Can you work these out from the model? Positions are in its coordinate system, mm. A direction names the side the tool comes from. Coordinates: 2 decimals unless noted, no trailing zeros. Order: outer loops, then holes, each group sorted by start corner. A loop starts at its lowest first (then second) coordinate and runs counter-clockwise, first axis right, second up. Notation, with made-up numbers: (59, -38) -> (109, -38) arc R12 ccw to (109, -21) -> close; hole circle Ø8 at (53, 46.5). An arc over 180 degrees is marked (long way). Answer as CSV lines item,"result".
from build123d import *

# Parameters (mm, degrees)
SKETCH_1_W       = 26.1
SKETCH_1_H       = 45.1
SKETCH_1_R       = 1
EXTRUDE_1_DEPTH  = 1.6
EXTRUDE_2_DEPTH  = 1.8
SKETCH_3_W       = 11
SKETCH_3_H       = 1
EXTRUDE_3_DEPTH  = 3
FILLET_1_R       = 0.5
SKETCH_4_W       = 8.1
SKETCH_4_H       = 8.1
EXTRUDE_4_DEPTH  = 2
SKETCH_5_R       = 4
EXTRUDE_5_DEPTH  = 4.8
SKETCH_6_R       = 5
EXTRUDE_6_DEPTH  = 2.7
SKETCH_7_W       = 12.5
SKETCH_7_H       = 7.7
EXTRUDE_7_DEPTH  = 6
SKETCH_9_W       = 1.2
SKETCH_9_H       = 4.4
EXTRUDE_8_DEPTH  = 2.9
SKETCH_10_W      = 18.1
SKETCH_10_H      = 25.5
EXTRUDE_9_DEPTH  = 0.8
SKETCH_11_W      = 15.86
SKETCH_11_H      = 17.74
EXTRUDE_10_DEPTH = 2.3
SKETCH_12_W      = 0.88
SKETCH_12_H      = 2
EXTRUDE_11_DEPTH = 0.8


with BuildPart() as part:
    # 草图1 → 凸台-拉伸1 (new body)
    with BuildSketch(Plane(origin=(0, 0, 0), x_dir=(1, 0, 0), z_dir=(0, 1, 0))):
        Rectangle(SKETCH_1_W, SKETCH_1_H)
        with Locations((-11.05, 20.55)):
            Circle(SKETCH_1_R, mode=Mode.SUBTRACT)
        with Locations((11.05, 20.55)):
            Circle(SKETCH_1_R, mode=Mode.SUBTRACT)
        with Locations((-11.05, -20.55)):
            Circle(SKETCH_1_R, mode=Mode.SUBTRACT)
        with Locations((11.05, -20.55)):
            Circle(SKETCH_1_R, mode=Mode.SUBTRACT)
    extrude(amount=EXTRUDE_1_DEPTH)

    # 草图2 → 凸台-拉伸2 (add)
    with BuildSketch(Plane(origin=(0, 1.6, 0), x_dir=(1, 0, 0), z_dir=(0, 1, 0))):
        Polygon((-7.05, 6.15), (7.95, 6.15), (7.95, 20.35), (-1.45, 20.35), (-2.75, 20.95), (-7.05, 20.95), align=None)
    extrude(amount=EXTRUDE_2_DEPTH)

    # 草图3 → 凸台-拉伸3 (add)
    with BuildSketch(Plane(origin=(0, 0, -20.35), x_dir=(-1, 0, 0), z_dir=(0, 0, -1))):
        with Locations((-1.65, 2.8)):
            Rectangle(SKETCH_3_W, SKETCH_3_H)
    extrude(amount=EXTRUDE_3_DEPTH)

    # 圆角1
    fillet_1_edges = [part.edges().sort_by_distance(p)[0] for p in [
        (-3.85, 2.8, -23.35),
        (7.15, 2.8, -23.35),
        (13.05, 0.8, -22.55),
        (13.05, 0.8, 22.55),
        (-13.05, 0.8, 22.55),
        (-13.05, 0.8, -22.55),
    ]]
    fillet(fillet_1_edges, radius=FILLET_1_R)

    # 草图4 → 凸台-拉伸4 (add)
    with BuildSketch(Plane(origin=(0, 3.4, 0), x_dir=(1, 0, 0), z_dir=(0, 1, 0))):
        with Locations((1, 10.2)):
            Rectangle(SKETCH_4_W, SKETCH_4_H)
    extrude(amount=EXTRUDE_4_DEPTH)

    # 草图5 → 凸台-拉伸5 (add)
    with BuildSketch(Plane(origin=(0, 5.4, 0), x_dir=(1, 0, 0), z_dir=(0, 1, 0))):
        with Locations((1, 10.2)):
            Circle(SKETCH_5_R)
    extrude(amount=EXTRUDE_5_DEPTH)

    # 草图6 → 凸台-拉伸6 (add)
    with BuildSketch(Plane(origin=(0, 10.2, 0), x_dir=(1, 0, 0), z_dir=(0, 1, 0))):
        with Locations((1, 10.2)):
            Circle(SKETCH_6_R)
    extrude(amount=EXTRUDE_6_DEPTH)

    # 草图7 → 凸台-拉伸7 (add)
    with BuildSketch(Plane.XZ):
        with Locations((0.3, -18.5)):
            Rectangle(SKETCH_7_W, SKETCH_7_H)
    extrude(amount=EXTRUDE_7_DEPTH)

    # 草图9 → 凸台-拉伸8 (add)
    with BuildSketch(Plane.XZ):
        with Locations((7.15, -19.35)):
            Rectangle(SKETCH_9_W, SKETCH_9_H)
        with Locations((-6.55, -19.35)):
            Rectangle(SKETCH_9_W, SKETCH_9_H)
    extrude(amount=EXTRUDE_8_DEPTH)

    # 草图10 → 凸台-拉伸9 (add)
    with BuildSketch(Plane.XZ):
        with Locations((0, 9.8)):
            Rectangle(SKETCH_10_W, SKETCH_10_H)
    extrude(amount=EXTRUDE_9_DEPTH)

    # 草图11 → 凸台-拉伸10 (add)
    with BuildSketch(Plane.XZ.offset(0.8)):
        with Locations((-0.05, 6.99)):
            Rectangle(SKETCH_11_W, SKETCH_11_H)
    extrude(amount=EXTRUDE_10_DEPTH)

    # 草图12 → 凸台-拉伸11 (add)
    with BuildSketch(Plane.XZ):
        with Locations((-11.46, 16.55)):
            Rectangle(SKETCH_12_W, SKETCH_12_H)
        with Locations((-11.46, 13.55)):
            Rectangle(SKETCH_12_W, SKETCH_12_H)
        with Locations((-11.46, 10.55)):
            Rectangle(SKETCH_12_W, SKETCH_12_H)
        with Locations((-11.46, 7.55)):
            Rectangle(SKETCH_12_W, SKETCH_12_H)
        with Locations((-11.46, 4.55)):
            Rectangle(SKETCH_12_W, SKETCH_12_H)
    extrude(amount=EXTRUDE_11_DEPTH)


solid = part.part
Q1. For P1, Ø3, axis at y = 3.5, z = 11, coming from the +X side; P2, Ø4, axis at x = 2.5, y = 10, coming from the +Z side; P3, Ø0.9, axis at y = 3, z = -13.5, coming from the -X side; P4, Ø1.6, axis at y = 4.5, z = -12, coming from the -X side, each with a flat end and sliding along its axis, tell me the tip position at first contact or that it passes through.
Solution:
P1,"through"
P2,"z = -5.2"
P3,"x = -7.05"
P4,"x = -3.05"
Q2. Imagine slicing it at B-B (z = 20.55). List the corners of the cut face in (x, y) for me.
Solution:
outline,"(-13.05, 0) -> (-12.05, 0) -> (-12.05, 1.6) -> (-13.05, 1.6) -> close; (-10.05, 0) -> (-9.05, 0) -> (-9.05, -0.8) -> (9.05, -0.8) -> (9.05, 0) -> (10.05, 0) -> (10.05, 1.6) -> (-10.05, 1.6) -> close; (12.05, 0) -> (13.05, 0) -> (13.05, 1.6) -> (12.05, 1.6) -> close"
Q3. If I drill on line 1 (Z direction, x = -11.05, y = 1.1); line 2 (X direction, y = 0.75, z = -20.55); line 3 (Y direction, x = -4.5, z = -7), over which ranges is the centre line in solid material (lowest first)?
Solution:
line 1,"-22.55 to -21.55, -19.55 to 19.55, 21.55 to 22.55"
line 2,"-13.05 to -12.05, -10.05 to 10.05, 12.05 to 13.05"
line 3,"0 to 3.4"
Q4. Which directions (+Z, -Z, +X, -X, +Y, -Y) give clear straight access to the entire face, cutting with the end or side of a thin tool? Please do faces 4 (the flat face through (2, 3.3, -22)), 5 (the flat face through (5.05, 4, -10)), 6 (the flat face through (0, -2, 15.86)), 7 (the flat face through (-11.5, -0.8, 13.6)).
Solution:
face 4,"-Z, +X, +Y"
face 5,"+Z, -Z, +X"
face 6,"+Z, +X, -X, -Y"
face 7,"+Z, -Z, -X, -Y"
Q5. We'd pull the mould along Z, two halves only. Please class faces 1 (the cylindrical face through (11.51, 0.79, -19.66)), 2 (the flat face through (7.95, 2, -13)), 3 (the cylindrical face through (0.349, 11.531, -15.157)): pulls with the +Z half, pulls with the -Z half, needs draft (parallel to the pull), parting line crosses it, or undercut.
Solution:
face 1,"undercut"
face 2,"needs draft"
face 3,"parting line crosses it"
Q6. Imagine slicing it at A-A (x = 11.05). List the corners of the cut face in (y, z) for me.
Solution:
outline,"(0, -22.55) -> (1.6, -22.55) -> (1.6, -21.55) -> (0, -21.55) -> close; (0, -19.55) -> (1.6, -19.55) -> (1.6, 19.55) -> (0, 19.55) -> close; (0, 21.55) -> (1.6, 21.55) -> (1.6, 22.55) -> (0, 22.55) -> close"
Q7. Imagine slicing it at C-C (z = -10.2). List the corners of the cut face in (x, y) for me.
Solution:
outline,"(-13.05, 0) -> (13.05, 0) -> (13.05, 1.6) -> (7.95, 1.6) -> (7.95, 3.4) -> (5.05, 3.4) -> (5.05, 5.4) -> (5, 5.4) -> (5, 10.2) -> (6, 10.2) -> (6, 12.9) -> (-4, 12.9) -> (-4, 10.2) -> (-3, 10.2) -> (-3, 5.4) -> (-3.05, 5.4) -> (-3.05, 3.4) -> (-7.05, 3.4) -> (-7.05, 1.6) -> (-13.05, 1.6) -> close"
